The listing builds one solid part. Answer for the finished solid, in the listing's coordinates (mm). Face numbers are marked on the shaded views. Give positions to 0.01 mm unless a question says otherwise; leave off trailing zeros. Write each loop counter-clockwise with the first axis right and the second up, starting at its lowest first coordinate (ties: lowest second). Pieces come first, ordered by that corner, then holes. Notation, with made-up numbers: (-19, 78.5) -> (27, 78.5) arc R33 cw to (27, 108.5) -> close; hole circle Ø4 at (51, 31.25). An arc over 180 degrees is marked (long way). Put each result on its own line as item: value. Start each with the question number.
1) A cutting plane is placed at B-B (y = 44.45). Write down the section's boundary in (x, z), then the cut area to 3 significant figures.
2) A cutting plane is placed at D-D (y = 11.5). Write down the section's boundary in (x, z), then the cut area to 3 significant figures.
3) A cutting plane is placed at C-C (z = -120). Write down the section's boundary in (x, y) (3 decimals).
4) Find the intervals of material crossed by line 1 along Z through (x, y) = (20, 44); line 2 along Y through (x, z) = (15, -19); line 3 along Y through (x, z) = (8, -19), in increasing order. Write a range as from..to.
5) A cutting plane is placed at A-A (x = 13). Write down the section's boundary in (y, z).
6) For a pull along X with two mould halves and no side action, classify the marked faces 1, 2 and 3 as released by +X, released by -X, zero draft, split by the parting line, or undercut.
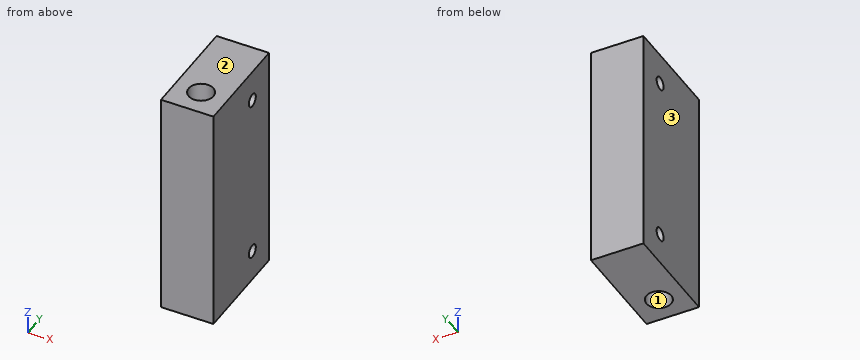
from build123d import *

# Parameters (mm, degrees)
SKETCH1_W           = 31.75
SKETCH1_H           = 63.5
SKETCH1_R           = 7.5
BOSS_EXTRUDE1_DEPTH = 139.7
SKETCH2_R           = 3.96875
CUT_EXTRUDE1_DEPTH  = 139.7


with BuildPart() as part:
    # Sketch1 → Boss-Extrude1 (new body)
    with BuildSketch(Plane.XY):
        with Locations((15.875, 31.75)):
            Rectangle(SKETCH1_W, SKETCH1_H)
        with Locations((15.875, 15.875)):
            Circle(SKETCH1_R, mode=Mode.SUBTRACT)
    extrude(amount=-BOSS_EXTRUDE1_DEPTH)

    # Sketch2 → Cut-Extrude1 (cut)
    with BuildSketch(Plane(origin=(31.75, 0, 0), x_dir=(0, 0, -1), z_dir=(1, 0, 0))):
        with Locations((19.05, 44.45)):
            Circle(SKETCH2_R)
        with Locations((120.65, 44.45)):
            Circle(SKETCH2_R)
    extrude(amount=-CUT_EXTRUDE1_DEPTH, mode=Mode.SUBTRACT)


solid = part.part
Reply:
1. outline: (0, -139.7) -> (31.75, -139.7) -> (31.75, -124.62) -> (0, -124.62) -> close; (0, -116.68) -> (31.75, -116.68) -> (31.75, -23.02) -> (0, -23.02) -> close; (0, -15.08) -> (31.75, -15.08) -> (31.75, 0) -> (0, 0) -> close
1. area: 3,930 mm2
2. outline: (0, -139.7) -> (9.78, -139.7) -> (9.78, 0) -> (0, 0) -> close; (21.97, -139.7) -> (31.75, -139.7) -> (31.75, 0) -> (21.97, 0) -> close
2. area: 2,730 mm2
3. outline: (0, 0) -> (31.75, 0) -> (31.75, 40.535) -> (0, 40.535) -> close; (0, 48.365) -> (31.75, 48.365) -> (31.75, 63.5) -> (0, 63.5) -> close; hole circle Ø15 at (15.875, 15.875)
4. line 1: z = -139.7..-124.59, -116.71..-22.99, -15.11..0
4. line 2: y = 0..8.43, 23.32..40.48, 48.42..63.5
4. line 3: y = 0..40.48, 48.42..63.5
5. outline: (0, -139.7) -> (8.95, -139.7) -> (8.95, 0) -> (0, 0) -> close; (22.8, -139.7) -> (63.5, -139.7) -> (63.5, 0) -> (22.8, 0) -> close; hole circle Ø7.94 at (44.45, -120.65); hole circle Ø7.94 at (44.45, -19.05)
6. face 1: undercut
6. face 2: zero draft
6. face 3: released by -X
